Input: dimensioned drawing with shaded views. Units: mm. Origin: part minimum x, y, z. Give positions to 0.01 mm unless a question says otherwise; leave off trailing zeros. Order: outer loops, then holes, each group sorted by start corner. A loop starts at its lowest first (then second) coordinate and runs counter-clockwise, first axis right, second up.
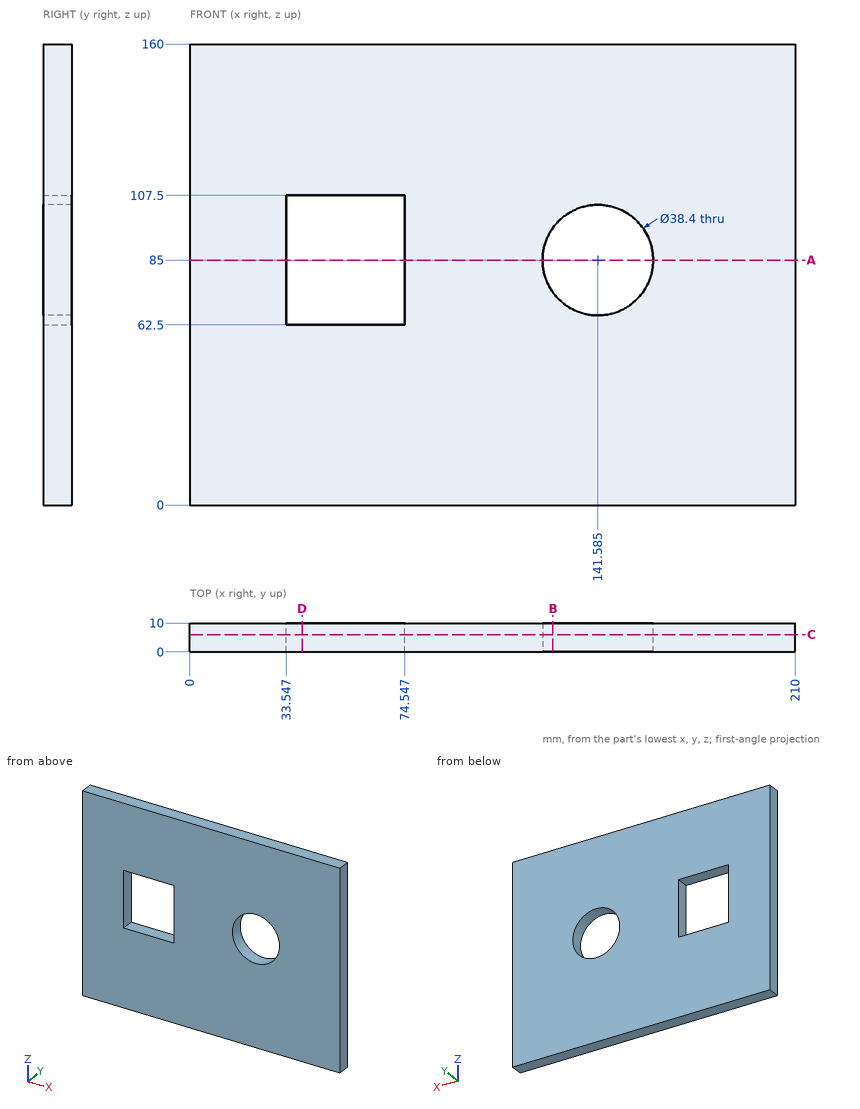
1) Section query C-C, the plane y = 6. Return the cut outline in (x, z) (1 decimal).
Report:
outline: (0, 0) - (210, 0) - (210, 160) - (0, 160) - close; hole (33.5, 62.5) - (74.5, 62.5) - (74.5, 107.5) - (33.5, 107.5) - close; hole circle Ø38.4 at (141.6, 85)
2) Section query A-A, the plane z = 85. Return the cut outline in (x, y) (1 decimal), and give its area (3 significant figures).
Report:
outline: (0, 0) - (33.5, 0) - (33.5, 10) - (0, 10) - close; (74.5, 0) - (122.4, 0) - (122.4, 10) - (74.5, 10) - close; (160.8, 0) - (210, 0) - (210, 10) - (160.8, 10) - close
area: 1,310 mm2
3) Section query B-B, the plane x = 126. Return the cut outline in (y, z), and give its area (3 significant figures).
Report:
outline: (0, 0) - (10, 0) - (10, 73.79) - (0, 73.79) - close; (0, 96.21) - (10, 96.21) - (10, 160) - (0, 160) - close
area: 1,380 mm2
4) Material intervals for L1, parallel to X at y = 4.75, z = 85 (1 decimal); L2, parallel to X at y = 4, z = 101 (1 decimal); L3, parallel to Z at x = 47, y = 6.25, sorted ascending.
Report:
L1: x = 0 to 33.5, 74.5 to 122.4, 160.8 to 210
L2: x = 0 to 33.5, 74.5 to 131, 152.2 to 210
L3: z = 0 to 62.5, 107.5 to 160
5) Section query D-D, the plane x = 39. Return the cut outline in (y, z), and give its area (3 significant figures).
Report:
outline: (0, 0) - (10, 0) - (10, 62.5) - (0, 62.5) - close; (0, 107.5) - (10, 107.5) - (10, 160) - (0, 160) - close
area: 1,150 mm2
